```python
from build123d import *

# Parameters (mm, degrees)
SKETCH_1_W          = 226
SKETCH_1_H          = 42
EXTRUDE_1_DEPTH     = 9.5
SKETCH_6_W          = 16
SKETCH_6_H          = 9.5
EXTRUDE_4_DEPTH     = 15
FILLET_1_R          = 3
SKETCH_7_R          = 1.9
CUT_EXTRUDE_1_DEPTH = 234.270765421
SKETCH_9_R          = 11.1
CUT_EXTRUDE_2_DEPTH = 10
SKETCH_11_R         = 4
CUT_EXTRUDE_4_DEPTH = 4


with BuildPart() as part:
    # 草图1 → 凸台-拉伸1 (new body)
    with BuildSketch(Plane(origin=(0, 0, 0), x_dir=(1, 0, 0), z_dir=(0, 1, 0))):
        with Locations((113, 21)):
            Rectangle(SKETCH_1_W, SKETCH_1_H)
    extrude(amount=EXTRUDE_1_DEPTH)

    # 草图6 → 凸台-拉伸4 (add)
    with BuildSketch(Plane(origin=(0, 0, -42), x_dir=(-1, 0, 0), z_dir=(0, 0, -1))):
        with Locations((-8, 4.75)):
            Rectangle(SKETCH_6_W, SKETCH_6_H)
        with Locations((-218, 4.75)):
            Rectangle(SKETCH_6_W, SKETCH_6_H)
    extrude(amount=EXTRUDE_4_DEPTH)

    # 圆角1
    fillet_1_edges = [part.edges().sort_by_distance(p)[0] for p in [
        (16, 4.75, -57),
        (210, 4.75, -57),
    ]]
    fillet(fillet_1_edges, radius=FILLET_1_R)

    # 草图7 → 切除-拉伸1 (cut, through all)
    with BuildSketch(Plane(origin=(0, 9.5, 0), x_dir=(1, 0, 0), z_dir=(0, 1, 0))):
        with Locations(Location((21, 34, 0), (0, 0, 270))):
            Circle(SKETCH_7_R)
        with Locations(Location((37, 8, 0), (0, 0, 270))):
            Circle(SKETCH_7_R)
        with Locations(Location((189, 8, 0), (0, 0, 270))):
            Circle(SKETCH_7_R)
        with Locations(Location((205, 34, 0), (0, 0, 270))):
            Circle(SKETCH_7_R)
    extrude(amount=-CUT_EXTRUDE_1_DEPTH, mode=Mode.SUBTRACT)

    # 草图9 → 切除-拉伸2 (cut)
    with BuildSketch(Plane(origin=(0, 9.5, 0), x_dir=(1, 0, 0), z_dir=(0, 1, 0))):
        with Locations(Location((113, 21, 0), (0, 0, 270))):
            Circle(SKETCH_9_R)
    extrude(amount=-CUT_EXTRUDE_2_DEPTH, mode=Mode.SUBTRACT)

    # 草图11 → 切除-拉伸4 (cut)
    with BuildSketch(Plane.XZ):
        with Locations(Location((37, -8, 0), (0, 0, 270))):
            Circle(SKETCH_11_R)
        with Locations(Location((21, -34, 0), (0, 0, 270))):
            Circle(SKETCH_11_R)
        with Locations(Location((189, -8, 0), (0, 0, 270))):
            Circle(SKETCH_11_R)
        with Locations(Location((205, -34, 0), (0, 0, 270))):
            Circle(SKETCH_11_R)
    extrude(amount=-CUT_EXTRUDE_4_DEPTH, mode=Mode.SUBTRACT)


solid = part.part
```
Here's how the part is built. I have some questions about the finished solid (model axes, mm). A direction names the side the tool comes from. Give positions to 0.01 mm unless a question says otherwise; leave off trailing zeros. Order: outer loops, then holes, each group sorted by start corner. A loop starts at its lowest first (then second) coordinate and runs counter-clockwise, first axis right, second up. Notation, with made-up numbers: M -19.75,87.25 L -4.75,87.25 A25 cw -4.75,99.25 Z; hole C -35,63 d6. An arc over 180 degrees is marked long. Use a Markdown table: item, result. Add a question column.
1. For pin 1 Ø2.5 at (x, z) = (21, -34) entering from +Y; pin 2 Ø3 at (x, y) = (73, 6) entering from -Z, each with a flat end and sliding along its axis, tell me the tip position at first contact or that it passes through.
2. On a 3-axis mill with a long thin cutter (end or side, diameter ignored), from which of +Z, -Z, +X, -X, +Y, -Y can I reach the whole of each face in a straight line? I mean faces 4 (the flat face through (210, 5, -48)), 5 (the flat face through (20, 4, -36)), 6 (the cylindrical face through (35.145, 6.788, -8.412)). Say none if no direction works.
3. If we mould it in two halves opening along Z, with no side actions, what happens to faces 1 (the flat face through (111, 5, 0)), 2 (the cylindrical face through (208.966, 1.972, -33.479)), 3 (the flat face through (16, 5, -48))? For each: +Z half, -Z half, draft (parallel to the pull), parting line (faces both ways), or undercut.
4. Suppose I cut it at C-C (z = -8). List the corners of the cut face in (x, y) for me, and give its area (3 significant figures).
5. Suppose I cut it at B-B (x = 113). List the corners of the cut face in (y, z) for me.
6. Suppose I cut it at A-A (z = -21). List the corners of the cut face in (x, y) for me, and give its area (3 significant figures).
7. I need wall thicknesses on probe 1 along X at (y, z) = (7.3, -34); probe 2 along X at (y, z) = (3.5, -21); probe 3 along X at (y, z) = (5, -50). Which ranges of each line are inside material? Lowest first, please. Write a range as from..to.
8. Suppose I cut it at D-D (y = 2.5). List the corners of the cut face in (x, z) for me, and give its area (3 significant figures).
Results list:
| question | item | result |
|---|---|---|
| 1 | pin 1 | passes through |
| 1 | pin 2 | stops at z = -42 |
| 2 | face 4 | -Z, +Y, -Y |
| 2 | face 5 | -Y |
| 2 | face 6 | +Y, -Y |
| 3 | face 1 | +Z half |
| 3 | face 2 | undercut |
| 3 | face 3 | draft |
| 4 | outline | M 0,0 L 33,0 L 33,4 L 35.1,4 L 35.1,9.5 L 0,9.5 Z; M 38.9,4 L 41,4 L 41,0 L 185,0 L 185,4 L 187.1,4 L 187.1,9.5 L 38.9,9.5 Z; M 190.9,4 L 193,4 L 193,0 L 226,0 L 226,9.5 L 190.9,9.5 Z |
| 4 | area | 2,040 mm² |
| 5 | outline | M 0,-42 L 9.5,-42 L 9.5,-32.1 L 0,-32.1 Z; M 0,-9.9 L 9.5,-9.9 L 9.5,0 L 0,0 Z |
| 6 | outline | M 0,0 L 101.9,0 L 101.9,9.5 L 0,9.5 Z; M 124.1,0 L 226,0 L 226,9.5 L 124.1,9.5 Z |
| 6 | area | 1,940 mm² |
| 7 | probe 1 | x = 0..19.1, 22.9..203.1, 206.9..226 |
| 7 | probe 2 | x = 0..101.9, 124.1..226 |
| 7 | probe 3 | x = 0..16, 210..226 |
| 8 | outline | M 0,-57 L 13,-57 A3 ccw 16,-54 L 16,-42 L 210,-42 L 210,-54 A3 ccw 213,-57 L 226,-57 L 226,0 L 0,0 Z; hole C 21,-34 d8; hole C 37,-8 d8; hole C 113,-21 d22.2; hole C 189,-8 d8; hole C 205,-34 d8 |
| 8 | area | 9,380 mm² |
